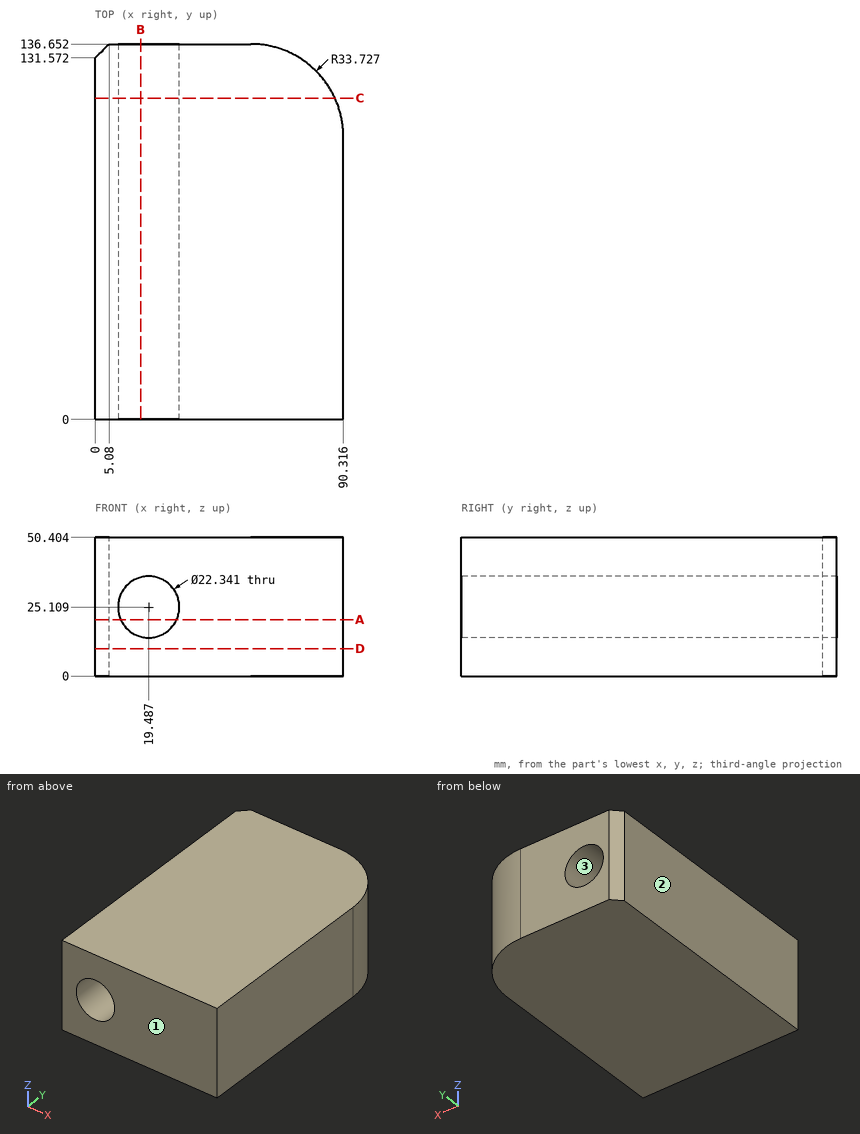
Print and shaded views of the part. All mm, measured from the part's lowest x, y and z. Coordinates: 2 decimals unless noted, no trailing zeros. Order: outer loops, then holes, each group sorted by start corner. A loop starts at its lowest first (then second) coordinate and runs counter-clockwise, first axis right, second up. Notation, with made-up numbers: (-16, -38) - (36, -38) arc R14 ccw to (36, -18) - close; hole circle Ø6 at (-40, 50). An arc over 180 degrees is marked (long way). Return JSON: item names as keys, results as strings. Group by question number.
Item 1: Cut at C-C (y = 117). List the corners of the cut face in (x, z) (1 decimal).
Item 2: Drill centre lines: probe 1 along X at (y, z) = (101.5, 28) (1 decimal); probe 2 along X at (y, z) = (75, 24) (1 decimal); probe 3 along Y at (x, z) = (58, 16.5). Where is each one in solid material? Low to high. Write a range as from..to.
Item 3: Cut at A-A (z = 20.5). List the corners of the cut face in (x, y) (1 decimal), plus the area to 3 significant figures.
Item 4: Pin check, flat tips, straight feed: pin 1 (4 mm diameter, centred on x = 67, z = 35, fed in from +Y); pin 2 (4 mm diameter, centred on x = 77, z = 37, fed in from +Y) (1 decimal). Stop position of each tip, or through.
Item 5: Pull direction X, two halves, no side cores. Call the marked faces 1, 2 and 3: pulls with the +X half, pulls with the -X half, needs draft (parallel to the pull), parting line crosses it, or undercut.
Item 6: Cut at B-B (x = 16.5). List the corners of the cut face in (y, z) (1 decimal), plus the area to 3 significant figures.
Item 7: Cut at D-D (z = 10). List the corners of the cut face in (x, y) (1 decimal).
Check values:
{
 "1": {"outline": "(0, 0) - (87.2, 0) - (87.2, 50.4) - (0, 50.4) - close; hole circle Ø22.3 at (19.5, 25.1)"},
 "2": {"probe 1": "x = 0..8.7, 30.3..90.3", "probe 2": "x = 0..8.4, 30.6..90.3", "probe 3": "y = 0..136.62"},
 "3": {"outline": "(0, 0) - (9.3, 0) - (9.3, 136.7) - (5.1, 136.7) - (0, 131.6) - close; (29.7, 0) - (90.3, 0) - (90.3, 102.9) arc R33.7 ccw to (56.6, 136.7) - (29.7, 136.7) - close", "area": "9,300 mm2"},
 "4": {"pin 1": "stops at y = 135.59", "pin 2": "stops at y = 131.2"},
 "5": {"face 1": "needs draft", "face 2": "pulls with the -X half", "face 3": "undercut"},
 "6": {"outline": "(0, 0) - (136.7, 0) - (136.7, 14.3) - (0, 14.3) - close; (0, 35.9) - (136.7, 35.9) - (136.7, 50.4) - (0, 50.4) - close", "area": "3,950 mm2"},
 "7": {"outline": "(0, 0) - (90.3, 0) - (90.3, 102.9) arc R33.7 ccw to (56.6, 136.7) - (5.1, 136.7) - (0, 131.6) - close"}
}
